Job drawing, mm, ordinate dimensions from the low corner. One solid piece. A direction names the side the tool comes from. Coordinates: 2 decimals unless noted, no trailing zeros. Order: outer loops, then holes, each group sorted by start corner. A loop starts at its lowest first (then second) coordinate and runs counter-clockwise, first axis right, second up. Notation, with made-up numbers: (59.25, 20.25) - (74.25, 20.25) arc R13 ccw to (74.25, 30.25) - close; hole circle Ø3 at (-2, 6). An arc over 180 degrees is marked (long way). Return JSON: item names as keys, results as strings.
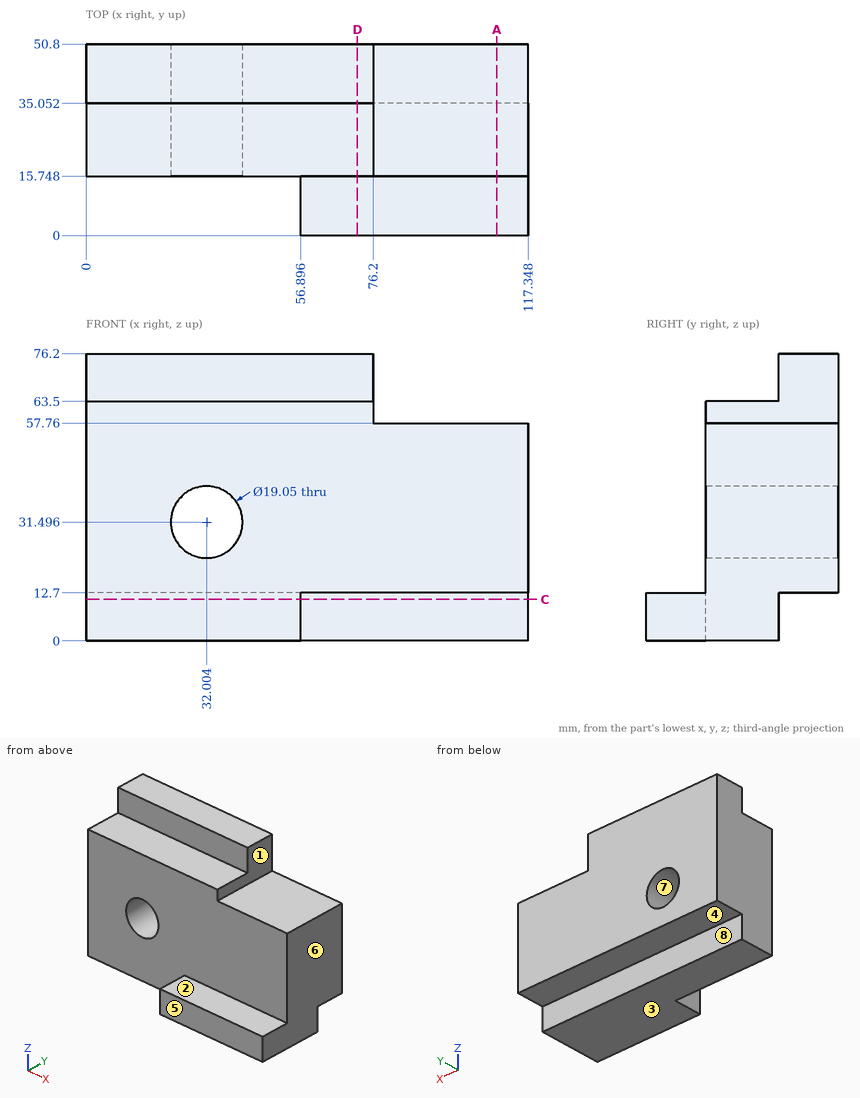
1. Cut at C-C on z = 11. Give the cut face in (x, y).
Check values:
{"outline": "(0, 15.75) - (56.9, 15.75) - (56.9, 0) - (117.35, 0) - (117.35, 35.05) - (0, 35.05) - close"}
2. Cut at A-A on x = 109. Give the cut face in (y, z), plus the area to 3 significant figures.
Check values:
{"outline": "(0, 0) - (35.05, 0) - (35.05, 12.7) - (50.8, 12.7) - (50.8, 57.76) - (15.75, 57.76) - (15.75, 12.7) - (0, 12.7) - close", "area": "2,020 mm²"}
3. Tool access for the marked faces 1, 2, 3, 4 and 5: list every direction of +Z, -Z, +X, -X, +Y, -Y with a clear straight run to the whole face (end or side of a thin tool).
Check values:
{"face 1": "+Z, +X, +Y, -Y", "face 2": "+Z, +X, -X, -Y", "face 3": "-Z, +X, -X, +Y, -Y", "face 4": "-Z, +X, -X, +Y", "face 5": "+Z, -Z, +X, -X, -Y"}
4. Probe L1, parallel to Z at x = 78.5, y = 17; L2, parallel to Z at x = 110.5, y = 42.5; L3, parallel to Y at x = 27, z = 66. List the from-to ranges inside material, lowest first.
Check values:
{"L1": "0 to 57.76", "L2": "12.7 to 57.76", "L3": "35.05 to 50.8"}
5. Drop flat-ended pins along their axis: pin 1 (15 mm diameter, centred on y = 26.5, z = 66, fed in from +X); pin 2 (3 mm diameter, centred on x = 78.5, y = 42, fed in from +Z); pin 3 (12 mm diameter, centred on x = 62, y = 11.5, fed in from -Z); pin 4 (8 mm diameter, centred on x = 52.5, y = 39.5, fed in from -Z). Give the stop position or say it passes through.
Check values:
{"pin 1": "x = 76.2", "pin 2": "z = 57.76", "pin 3": "z = 0", "pin 4": "z = 12.7"}
6. Mould opens along X. For the marked faces 6, 7 and 8 say: pulls with the +X half, pulls with the -X half, needs draft (parallel to the pull), parting line crosses it, or undercut.
Check values:
{"face 6": "pulls with the +X half", "face 7": "undercut", "face 8": "needs draft"}
7. Cut at D-D on x = 72. Give the cut face in (y, z).
Check values:
{"outline": "(0, 0) - (35.05, 0) - (35.05, 12.7) - (50.8, 12.7) - (50.8, 76.2) - (35.05, 76.2) - (35.05, 63.5) - (15.75, 63.5) - (15.75, 12.7) - (0, 12.7) - close"}
